Autodesk Inventor part; units mm, degrees
ref_plane "YZ Plane" through (0, 0, 0) normal (1, 0, 0) x (0, 1, 0)
ref_plane "XZ Plane" through (0, 0, 0) normal (0, 1, 0) x (-1, 0, 0)
ref_plane "XY Plane" through (0, 0, 0) normal (0, 0, 1) x (1, 0, 0)
sketch "Sketch1" plane through (0, 0, 0) normal (0, 0, 1) x (1, 0, 0)
  line L0 (0, 0) -> (100, 0)
  line L1 (100, 0) -> (100, 15)
  line L2 (100, 15) -> (0, 15)
  line L3 (0, 15) -> (0, 0)
  line L4 (100, 0) -> (108, 0)
  line L5 (108, 0) -> (108, 25)
  line L6 (108, 25) -> (100, 25)
  line L7 (100, 25) -> (100, 0)
  dimension "d0" = 15
  dimension "d1" = 25
  dimension "d2" = 100
  dimension "d3" = 8
revolve "Revolution1" add sketch "Sketch1" angle 360 about axis through (0, 0, 0) along (1, 0, 0)
fillet "Fillet1" radius 3 1 edges at (100, -15, 0)
chamfer "Chamfer1" distance 2 angle 45 1 edges at (0, -15, 0)
sketch "Sketch2" plane through (0, 0, 0) normal (-1, 0, 0) x (0, 0, 1)
  point P0 (0, 0)
  point P1 (0, 0)
hole "Hole1" at (0, 0, 0) direction (1, 0, 0) diameter 6.647 depth 22.2 tip angle 118
sketch "Sketch3" plane through (108, 0, 0) normal (1, 0, 0) x (0, 0, -1)
  line L0 (-25, 2.5) -> (25, 2.5)
  line L1 (25, 2.5) -> (25, -2.5)
  line L2 (25, -2.5) -> (-25, -2.5)
  line L3 (-25, -2.5) -> (-25, 2.5)
  circle A0 centre (0, 0) radius 18
  circle A1 centre (0, 0) radius 25
  dimension "d16" = 50
  dimension "d17" = 50
  dimension "d18" = 25
  dimension "d19" = 5
  dimension "d20" = 2.5
extrude "Extrusion1" cut sketch "Sketch3" against normal blind 5 contours L0 A1 L3 | L0 A0 L2 A1 | A1 L2 L3 | L0 A0 L2 | A1 L2 A0 L0 | L0 L1 A1 | L1 L2 A1
equation "\"d17\" = d16"
properties part number "Top_Hinge Cylinder" material "Stainless Steel"
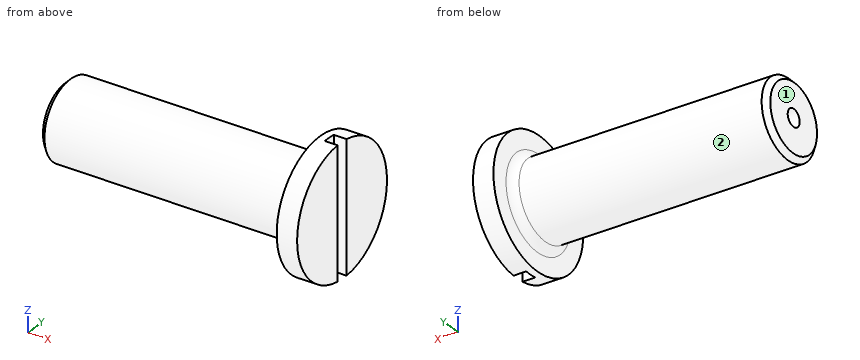
Source: CAD feature listing. Evaluate the final solid. Frame: model axes, mm. Face numbers are marked on the shaded views. A direction names the side the tool comes from. Round coordinates to 2 decimals unless told otherwise and drop trailing zeros. Loops run counter-clockwise (first coordinate to the right, second up) from the corner with the lowest first, then second, coordinate; pieces in that order, holes last. Notation, with made-up numbers: (17, 20) - (26, 20) arc R29 ccw to (26, 41) - close; hole circle Ø4 at (74.5, -39). An arc over 180 degrees is marked (long way). Write item = value, one per line. Start each with the question number.
(1) Section query A-A, the plane x = 90. Output: boundary loops of the cut face in (y, z).
(2) Section query B-B, the plane y = 20. Output: boundary loops of the cut face in (x, z), plus the area to 3 significant figures.
(3) Set-up query: the marked faces 1 and 2. Return all of +Z, -Z, +X, -X, +Y, -Y with unobstructed straight access to the full face (end or side cutting, diameter ignored); none if empty.
(4) Pin query (flat end, axial travel): pin 1 (10 mm diameter, centred on x = 52.5, z = -6, fed in from -Y); pin 2 (1 mm diameter, centred on x = 32.5, y = 9, fed in from -Z); pin 3 (5 mm diameter, centred on x = 49, y = 9, fed in from +Z). Return the tip coordinate at first contact, or that it passes through.
(5) Ray query, line 1 along Z through (x, y) = (7, 0); line 2 along X through (y, z) = (7, 17); line 3 along X through (y, z) = (1, 7.5). Return the intervals inside material, ascending. Write a range as from..to.
Conclusion:
q1.outline = circle Ø30 at (0, 0)
q2.outline = (100, -15) - (108, -15) - (108, 15) - (100, 15) - close
q2.area = 240 mm2
q3.face_1 = +Z, -Z, -X, +Y, -Y
q3.face_2 = -X
q4.pin_1 = -14.97
q4.pin_2 = -12.36
q4.pin_3 = 13.52
q5.line_1 = -15..-3.32, 3.32..15
q5.line_2 = 100..108
q5.line_3 = 0..103
